The listing builds one solid part. Answer for the finished solid, in the listing's coordinates (mm). Coordinates: 2 decimals unless noted, no trailing zeros. Loops run counter-clockwise (first coordinate to the right, second up) from the corner with the lowest first, then second, coordinate; pieces in that order, holes last. Notation, with made-up numbers: (-3.5, 6.5) - (11.5, 6.5) arc R22 cw to (11.5, 36.5) - close; hole circle Ø2 at (80, -27.5). An arc over 180 degrees is marked (long way). Return JSON: item names as keys, results as strings. Group by question number.
1. Each of these flat-tipped pins is pushed along its axis until it touches: P1, Ø1, axis at y = 7, z = -21.5, coming from the +X side; P2, Ø2, axis at x = 22.5, y = -2, coming from the +Z side; P3, Ø8, axis at x = 42.5, z = -15.5, coming from the -Y side. Where does it stop, or does it pass through?
2. Section A-A (y = 14.5) is taken. Write down the section's boundary in (x, z), and give its area (3 significant figures).
3. Find the intervals of material crossed by line 1 along X through (y, z) = (11, -16.5); line 2 along X through (y, z) = (-15, -26.5); line 3 along Y through (x, z) = (53, -19), in increasing order.
4. Section B-B (x = 18) is taken. Write down the section's boundary in (y, z), and give its area (3 significant figures).
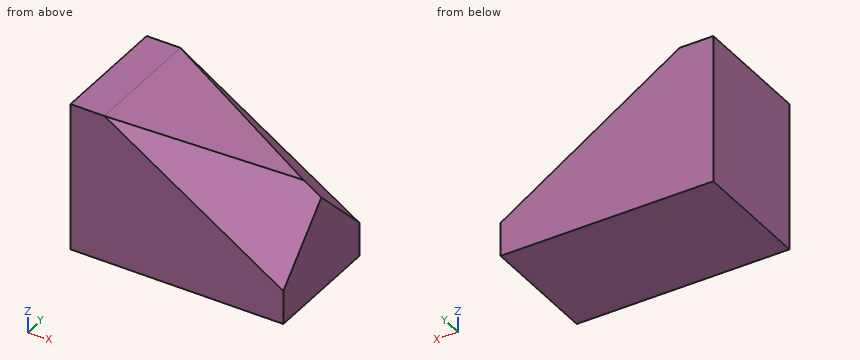
Autodesk Inventor part; units mm, degrees
ref_plane "工作平面1" through (10, 18, 0) normal (-0.4131, -0.644, -0.644) x (0.8417, 0, -0.54)
ref_plane "YZ Plane" through (0, 0, 0) normal (1, 0, 0) x (0, 1, 0)
ref_plane "XZ Plane" through (0, 0, 0) normal (0, 1, 0) x (-1, 0, 0)
sketch "草圖1" plane through (0, 0, 0) normal (0, 1, 0) x (-1, 0, 0)
  line L0 (0, 0) -> (-63, 0)
  line L1 (-63, 0) -> (-63, -44)
  line L2 (-63, -44) -> (0, -44)
  line L3 (0, -44) -> (0, 0)
  dimension "d0" = 63
  dimension "d1" = 44
extrude "擠出1" add sketch "草圖1" along normal mid plane 36
sketch "草圖2" plane through (0, 18, 0) normal (0, 1, 0) x (1, 0, 0)
  line L0 (0, 0) -> (63, 0)
  line L1 (10, 0) -> (63, 14)
  line L2 (63, 0) -> (63, 44)
  dimension "d4" = 10
  dimension "d5" = 30
extrude "擠出2" cut sketch "草圖2" against normal blind 40
sketch "草圖3" plane through (63, -18, -44) normal (1, 0, 0) x (0, 0, -1)
  line L0 (-30, 16) -> (-10, 36)
  line L1 (0, 36) -> (-44, 36)
  line L2 (-30, 36) -> (-30, 0)
  point P0 (-44, 18)
  dimension "d8" = 20
  dimension "d9" = 20
ref_plane "工作平面1" through (10, 18, 0) normal (-0.4131, -0.644, -0.644) x (0.8417, 0, -0.54)
sketch "草圖4" plane through (10, 18, 0) normal (-0.4131, -0.644, -0.644) x (0.8417, 0, -0.54)
  line L0 (-15.1543, -12.3218) -> (93.717, -12.3218)
  line L1 (93.717, -12.3218) -> (93.717, 28.8166)
  line L2 (93.717, 28.8166) -> (-15.1543, 28.8166)
  line L3 (-15.1543, 28.8166) -> (-15.1543, -12.3218)
  point P0 (-8.4169, 10.2941)
extrude "擠出3" cut sketch "草圖4" against normal blind 40
mirror "鏡射1" about plane through (0, 0, 0) normal (0, 1, 0) of "擠出3"
properties part number "24"
The answers:
{
 "1": {"P1": "stops at x = 61.76", "P2": "stops at z = -3.04", "P3": "stops at y = -17.4"},
 "2": {"outline": "(0, -44) - (63, -44) - (63, -30.5) - (19.27, -2.45) - (10, 0) - (0, 0) - close", "area": "2,040 mm2"},
 "3": {"line 1": "x = 0 to 46.63", "line 2": "x = 0 to 55.98", "line 3": "y = -9.41 to 9.41"},
 "4": {"outline": "(-18, -44) - (18, -44) - (18, -5.13) - (14.98, -2.11) - (-14.98, -2.11) - (-18, -5.13) - close", "area": "1,500 mm2"}
}
